Work out the finished part from the listing and answer in its coordinate system (mm). Face numbers are marked on the shaded views. A direction names the side the tool comes from. Round coordinates to 2 decimals unless told otherwise and drop trailing zeros. Loops run counter-clockwise (first coordinate to the right, second up) from the corner with the lowest first, then second, coordinate; pieces in that order, holes last. Notation, with made-up numbers: (47, 70.5) - (51, 70.5) arc R18 ccw to (51, 80.5) - close; hole circle Ø7 at (74.5, 88.5). An arc over 180 degrees is marked (long way). Use CSV: the item, a comma, the result in double quotes. Start each with the question number.
from build123d import *

# Parameters (mm, degrees)
PAD_DEPTH    = 15
SKETCH001_R  = 1.6
POCKET_DEPTH = 5


with BuildPart() as part:
    # Sketch → Pad (new body)
    with BuildSketch(Plane.XZ):
        Polygon((-3.1, 0), (-13.1, 0), (-13.1, 5), (13.1, 5), (13.1, 0), (3.1, 0), (3.1, 0.8), (-3.1, 0.8), align=None)
    extrude(amount=PAD_DEPTH)

    # Sketch001 (on Face3 of Pad) → Pocket (cut)
    with BuildSketch(Plane(origin=(0, 0, 5), x_dir=(-1, 0, 0), z_dir=(0, 0, 1))):
        with Locations((-8.1, 7.5)):
            Circle(SKETCH001_R)
        with Locations((8.1, 7.5)):
            Circle(SKETCH001_R)
    extrude(amount=-POCKET_DEPTH, mode=Mode.SUBTRACT)


solid = part.part
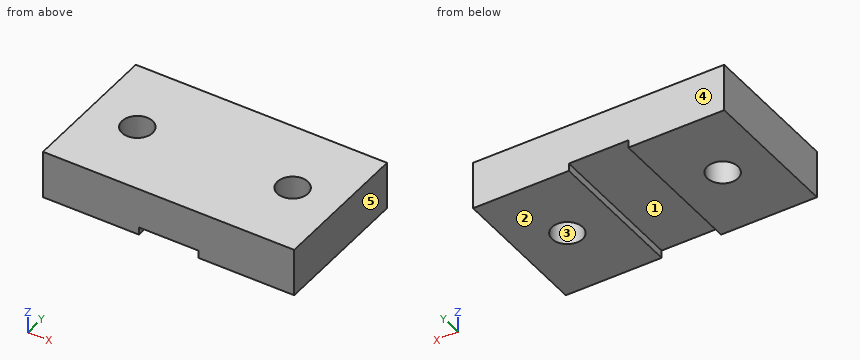
Item 1: A cutting plane is placed at B-B (z = 0.45). Determine the outline of the cut face in (x, y).
Item 2: Find the intervals of material crossed by probe 1 along X at (y, z) = (-7.5, 2.65); probe 2 along Y at (x, z) = (8.1, 2.3); probe 3 along X at (y, z) = (-8, 1.95), in increasing order. Write a range as [from, to].
Item 3: The mould has two halves that part along Y. Classify the marked faces 3, 4 and 5: pulls with the +Y half, pulls with the -Y half, needs draft (parallel to the pull), parting line crosses it, or undercut.
Item 4: A cutting plane is placed at D-D (y = -11). Determine the outline of the cut face in (x, z).
Item 5: A cutting plane is placed at C-C (x = -8.1). Determine the outline of the cut face in (y, z), plus the area to 3 significant figures.
Item 6: Which of the six approach directions +Z, -Z, +X, -X, +Y, -Y give full straight-line access (tool end or side, diameter ignored) to the marked faces 1 and 2?
Item 7: A cutting plane is placed at A-A (y = -7.5). Determine the outline of the cut face in (x, z), plus the area to 3 significant figures.
Item 8: This flat-tipped pin is pushed along its axis until it touches: pin 1 Ø1.5 at (x, z) = (8, 1) entering from +Y. Where does it stop, or does it pass through?
Result sheet:
1,outline,"(-13.1, -15) - (-3.1, -15) - (-3.1, 0) - (-13.1, 0) - close; (3.1, -15) - (13.1, -15) - (13.1, 0) - (3.1, 0) - close; hole circle Ø3.2 at (-8.1, -7.5); hole circle Ø3.2 at (8.1, -7.5)"
2,probe 1,"[-13.1, -9.7], [-6.5, 6.5], [9.7, 13.1]"
2,probe 2,"[-15, -9.1], [-5.9, 0]"
2,probe 3,"[-13.1, -9.62], [-6.58, 6.58], [9.62, 13.1]"
3,face 3,"undercut"
3,face 4,"pulls with the +Y half"
3,face 5,"needs draft"
4,outline,"(-13.1, 0) - (-3.1, 0) - (-3.1, 0.8) - (3.1, 0.8) - (3.1, 0) - (13.1, 0) - (13.1, 5) - (-13.1, 5) - close"
5,outline,"(-15, 0) - (-9.1, 0) - (-9.1, 5) - (-15, 5) - close; (-5.9, 0) - (0, 0) - (0, 5) - (-5.9, 5) - close"
5,area,"59.0 mm^2"
6,face 1,"-Z, +Y, -Y"
6,face 2,"-Z, +X, -X, +Y, -Y"
7,outline,"(-13.1, 0) - (-9.7, 0) - (-9.7, 5) - (-13.1, 5) - close; (-6.5, 0) - (-3.1, 0) - (-3.1, 0.8) - (3.1, 0.8) - (3.1, 0) - (6.5, 0) - (6.5, 5) - (-6.5, 5) - close; (9.7, 0) - (13.1, 0) - (13.1, 5) - (9.7, 5) - close"
7,area,"94.0 mm^2"
8,pin 1,"y = 0"
